Geometry check sheet. Reference: drawing and pictorial views, mm from the part's lowest x, y, z. A direction names the side the tool comes from. Round coordinates to 2 decimals unless told otherwise and drop trailing zeros. Write each loop counter-clockwise with the first axis right and the second up, starting at its lowest first coordinate (ties: lowest second). Pieces come first, ordered by that corner, then holes. Notation, with made-up numbers: (44, -37) -> (76, -37) arc R27 cw to (76, -16) -> close; hole circle Ø10 at (52, 40). An arc over 180 degrees is marked (long way). Write item = value, one per line.
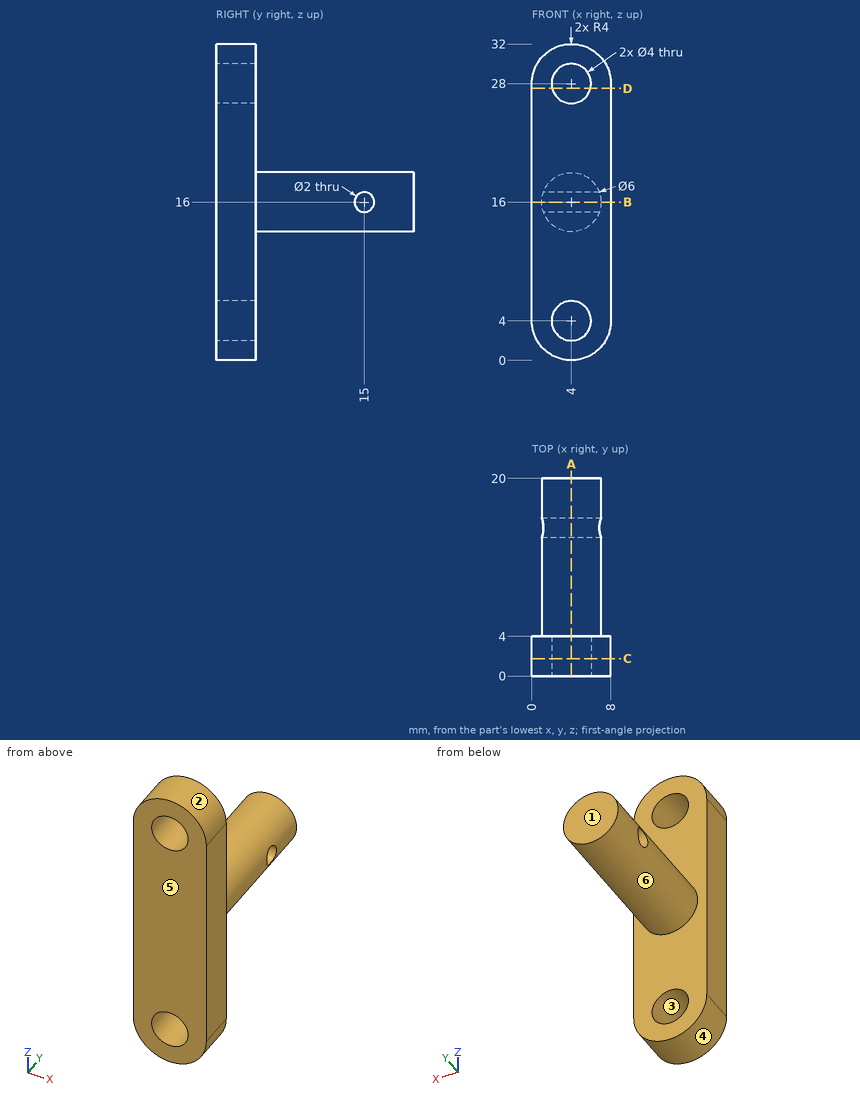
(1) Sectioned sample at A-A on x = 4. Enter the section's corners in (y, z).
Worked answers:
outline = (0, 0) -> (4, 0) -> (4, 2) -> (0, 2) -> close; (0, 6) -> (4, 6) -> (4, 13) -> (20, 13) -> (20, 19) -> (4, 19) -> (4, 26) -> (0, 26) -> close; (0, 30) -> (4, 30) -> (4, 32) -> (0, 32) -> close; hole circle Ø2 at (15, 16)
(2) Release check for a two-part mould opening along Z. For the marked faces 1, 2, 3 and 4 record: pulls with the +Z half, pulls with the -Z half, needs draft (parallel to the pull), parting line crosses it, or undercut.
Worked answers:
face_1 = needs draft
face_2 = pulls with the +Z half
face_3 = undercut
face_4 = pulls with the -Z half
(3) Sectioned sample at D-D on z = 27.5. Enter the section's corners in (x, y), then the cut area to 3 significant figures.
Worked answers:
outline = (0, 0) -> (2.06, 0) -> (2.06, 4) -> (0, 4) -> close; (5.94, 0) -> (8, 0) -> (8, 4) -> (5.94, 4) -> close
area = 16.5 mm²
(4) Go/stop test with flat-tipped pins: P1, Ø4, axis at x = 4, y = 9, coming from the -Z side; P2, Ø3, axis at x = 3, y = 17.5, coming from the +Z side; P3, Ø6, axis at y = 15, z = 12, coming from the -X side; P4, Ø1.2, axis at y = 15, z = 16, coming from the -X side. Record where each tip stops, or that it passes through.
Worked answers:
P1 = 13
P2 = 19
P3 = 1.17
P4 = through
(5) Access from +Z, -Z, +X, -X, +Y, -Y to the whole of each face (thin tool, end or side, straight path). Record for the marked faces 5 and 6.
Worked answers:
face_5 = +Z, -Z, +X, -X, -Y
face_6 = +Y
(6) Sectioned sample at B-B on z = 16. Enter the section's corners in (x, y).
Worked answers:
outline = (0, 0) -> (8, 0) -> (8, 4) -> (7, 4) -> (7, 14) -> (1, 14) -> (1, 4) -> (0, 4) -> close; (1, 16) -> (7, 16) -> (7, 20) -> (1, 20) -> close
(7) Sectioned sample at C-C on y = 1.75. Enter the section's corners in (x, z), then the cut area to 3 significant figures.
Worked answers:
outline = (0, 4) arc R4 ccw to (8, 4) -> (8, 28) arc R4 ccw to (0, 28) -> close; hole circle Ø4 at (4, 4); hole circle Ø4 at (4, 28)
area = 217 mm²
(8) Material ranges on L1, parallel to X at y = 2.1, z = 4; L2, parallel to Y at x = 2.5, z = 16; L3, parallel to Y at x = 7.25, z = 23.5, recorded low to high. Write a range as [from, to].
Worked answers:
L1 = [0, 2], [6, 8]
L2 = [0, 14], [16, 20]
L3 = [0, 4]
